Geometry: final body of the model. Coordinates: model frame, mm. A direction names the side the tool comes from. Give positions to 0.01 mm unless a question says otherwise; leave off trailing zeros. Order: outer loops, then holes, each group sorted by start corner. A loop starts at its lowest first (then second) coordinate and runs counter-clockwise, first axis right, second up. Notation, with made-up numbers: (87.5, 45) -> (92.5, 45) arc R30 cw to (92.5, 69) -> close; hole circle Ø6 at (58, -21). An arc over 180 degrees is marked (long way). Answer in a Markdown table with one row per item. Add a question column.
Q1. Pull-direction query (X, two-part tool) for faces 1 (the face through (23.846, 7.509, 4.437)), 2 (the face through (10, -10, 10)), 3 (the face through (-10.22, -8.21, 4.44)); classes: +X half, -X half, draft (parallel to the pull), parting line (faces both ways), or undercut.
Q2. Contact query for flat-ended pins moving along their axis: P1, Ø19.5, axis at x = 2.5, y = 1.5, coming from the +Z side; P2, Ø6, axis at y = 7.5, z = 0, coming from the -X side; P3, Ø1.6, axis at x = -0.5, z = 5, coming from the +Y side; P4, Ø7.5, axis at x = 0, y = 0, coming from the -Z side. Output: stop coordinate, or through.
Q3. Cut plane A-A on x = 0. Return the cut outline in (y, z), and give its area (3 significant figures).
Q4. Cut plane B-B on z = 7.75. Return the cut outline in (x, y), and give its area (3 significant figures).
Q5. Line query: line 1 along Y through (x, z) = (0, -2.3); line 2 along X through (y, z) = (0, -1); line 3 along Y through (x, z) = (-8, 2.25). Output: solid intervals per line, ascending. Write a range as from..to.
Q6. Set-up query: faces 4 (the face through (-15, 10, 4)), 5 (the face through (10, -17.16, 3.59)). Return all of +Z, -Z, +X, -X, +Y, -Y with unobstructed straight access to the full face (end or side cutting, diameter ignored); none if empty.
Q7. Cut plane C-C on y = 0. Count the separate pieces of the cut face and the enclosed holes in it, and give its area (3 significant figures).
from build123d import *

# Parameters (mm, degrees)
SKETCH_R          = 25
PAD_DEPTH         = 10
SKETCH001_R       = 28.5
PAD001_DEPTH      = 3
SKETCH002_R       = 4.25
SKETCH002_R_2     = 2.65
POCKET_DEPTH      = 10.501
POCKET_DEPTH_BACK = -2.501
FILLET_R          = 1
FILLET001_R       = 1
CHAMFER_SIZE      = 1
POCKET001_DEPTH   = 13.001


with BuildPart() as part:
    # Sketch → Pad (new body)
    with BuildSketch(Plane.XY):
        Circle(SKETCH_R)
        with BuildLine():
            ThreePointArc((17.347253, -6.023093), (21.799021, 0.111063), (17.133775, 6.08447))
            Line((15, 6.657422), (17.133775, 6.08447))
            Line((15, 14), (15, 6.657422))
            Line((-15, 14), (15, 14))
            Line((-15, 14), (-15, 6.657422))
            Line((-17.133775, 6.08447), (-15, 6.657422))
            ThreePointArc((-17.133775, 6.08447), (-21.799021, 0.111063), (-17.347253, -6.023093))
            Line((-17.347253, -6.023093), (-2.75, -10.5))
            Line((-2.75, -10.5), (2.75, -10.5))
            Line((17.347253, -6.023093), (2.75, -10.5))
        make_face(mode=Mode.SUBTRACT)
    extrude(amount=PAD_DEPTH)

    # Sketch001 (on Face12 of Pad) → Pad001 (join)
    with BuildSketch(Plane(origin=(0, 0, 0), x_dir=(1, 0, 0), z_dir=(0, 0, -1))):
        Circle(SKETCH001_R)
    extrude(amount=PAD001_DEPTH)

    # Sketch002 → Pocket (cut, two sides)
    with BuildSketch(Plane(origin=(0, 0, -0.5), x_dir=(1, 0, 0), z_dir=(0, 0, -1))) as pocket_sk:
        Circle(SKETCH002_R)
        with Locations((-15.75, 0)):
            Circle(SKETCH002_R_2)
        with Locations((15.75, 0)):
            Circle(SKETCH002_R_2)
    extrude(amount=-POCKET_DEPTH, mode=Mode.SUBTRACT)
    extrude(pocket_sk.sketch, amount=-POCKET_DEPTH_BACK, mode=Mode.SUBTRACT)

    # Fillet
    fillet_edges = [part.edges().sort_by_distance(p)[0] for p in [
        (15, 6.657422, 5),
        (15, 14, 5),
        (-15, 6.657422, 5),
        (-15, 14, 5),
        (-2.75, -10.5, 5),
        (2.75, -10.5, 5),
    ]]
    fillet(fillet_edges, radius=FILLET_R)

    # Fillet001
    fillet001_edges = [part.edges().sort_by_distance(p)[0] for p in [
        (0, 14, 10),
        (-15, 10.212165, 10),
        (-21.799021, 0.111063, 10),
        (-10.120283, -8.23957, 10),
        (0, -10.5, 10),
        (10.120283, -8.23957, 10),
        (21.799021, 0.111063, 10),
        (15, 10.212165, 10),
        (14.707107, 13.707107, 10),
        (15.206486, 6.815778, 10),
        (16.437223, 6.271505, 10),
        (-16.437223, 6.271505, 10),
        (-15.206486, 6.815778, 10),
        (-14.707107, 13.707107, 10),
        (-2.748344, -10.488951, 10),
        (2.748344, -10.488951, 10),
    ]]
    fillet(fillet001_edges, radius=FILLET001_R)

    # Chamfer
    chamfer_edges = [part.edges().sort_by_distance(p)[0] for p in [
        (-25, 0, 10),
    ]]
    chamfer(chamfer_edges, length=CHAMFER_SIZE)

    # Sketch003 (on Face1 of Chamfer) → Pocket001 (cut, through all)
    with BuildSketch(Plane.XY.offset(10)):
        with BuildLine():
            ThreePointArc((-7.124188, -14.225591), (-9.999095, -17.100498), (-7.124188, -19.975405))
            Line((-7.124188, -19.975405), (7.124188, -19.975405))
            ThreePointArc((7.124188, -19.975405), (9.999095, -17.100498), (7.124188, -14.225591))
            Line((-7.124188, -14.225591), (7.124188, -14.225591))
        make_face()
    extrude(amount=-POCKET001_DEPTH, mode=Mode.SUBTRACT)


solid = part.part
Completed:
| question | item | result |
|---|---|---|
| 1 | face 1 | parting line |
| 1 | face 2 | draft |
| 1 | face 3 | undercut |
| 2 | P1 | stops at z = 0 |
| 2 | P2 | stops at x = -28.14 |
| 2 | P3 | stops at y = 25 |
| 2 | P4 | passes through |
| 3 | outline | (-28.5, -3) -> (-19.98, -3) -> (-19.98, 10) -> (-24, 10) -> (-25, 9) -> (-25, 0) -> (-28.5, 0) -> close; (-14.23, -3) -> (-4.25, -3) -> (-4.25, 0) -> (-10.5, 0) -> (-10.5, 9) arc R1 ccw to (-11.5, 10) -> (-14.23, 10) -> close; (4.25, -3) -> (28.5, -3) -> (28.5, 0) -> (25, 0) -> (25, 9) -> (24, 10) -> (15, 10) arc R1 ccw to (14, 9) -> (14, 0) -> (4.25, 0) -> close |
| 3 | area | 324 mm² |
| 4 | outline | circle Ø50 at (0, 0); hole (-17.35, -6.02) -> (-2.89, -10.46) arc R1 ccw to (-2.6, -10.5) -> (2.6, -10.5) arc R1 ccw to (2.89, -10.46) -> (17.35, -6.02) arc R6.3 ccw to (17.13, 6.08) -> (15.74, 6.46) arc R1 cw to (15, 7.42) -> (15, 13) arc R1 ccw to (14, 14) -> (-14, 14) arc R1 ccw to (-15, 13) -> (-15, 7.42) arc R1 cw to (-15.74, 6.46) -> (-17.13, 6.08) arc R6.3 ccw to start; hole (-7.12, -19.98) -> (7.12, -19.98) arc R2.87 ccw to (7.12, -14.23) -> (-7.12, -14.23) arc R2.87 ccw to start |
| 4 | area | 1,030 mm² |
| 5 | line 1 | y = -28.5..-19.98, -14.23..-4.25, 4.25..28.5 |
| 5 | line 2 | x = -28.5..-18.4, -13.1..-4.25, 4.25..13.1, 18.4..28.5 |
| 5 | line 3 | y = -23.69..-19.84, -14.36..-8.89, 14..23.69 |
| 6 | face 4 | +Z |
| 6 | face 5 | +Z, -Z |
| 7 | separate pieces | 4 |
| 7 | enclosed holes | 0 |
| 7 | area | 176 mm² |
